```python
from build123d import *

# Parameters (mm, degrees)
F1_DEPTH = 18
F2_R     = 3
F3_R     = 3
F4_R     = 12
F5_R     = 0.5


with BuildPart() as f1:
    # F0 (on Top) → F1 (new body)
    with BuildSketch(Plane.XY):
        Polygon((-61.901969, -15.611527), (28.098031, -15.611527), (20.267047, 16.256898), (12.498162, 14.347861), (17.032125, -4.103242), (7.746533, -3.611527), (-6.571248, 54.655111), (-14.340133, 52.746074), (0, -5.611527), (-61.901969, -5.611527), align=None)
    extrude(amount=F1_DEPTH)

    # F2
    f2_edges = [f1.edges().sort_by_distance(p)[0] for p in [
        (12.498162, 14.347861, 9),
        (-6.571248, 54.655111, 9),
    ]]
    fillet(f2_edges, radius=F2_R)

    # F3
    f3_edges = [f1.edges().sort_by_distance(p)[0] for p in [
        (-61.901969, -5.611527, 9),
    ]]
    fillet(f3_edges, radius=F3_R)

    # F4
    f4_edges = [f1.edges().sort_by_distance(p)[0] for p in [
        (0, -5.611527, 9),
    ]]
    fillet(f4_edges, radius=F4_R)

    # F5
    f5_edges = [f1.edges().sort_by_distance(p)[0] for p in [
        (17.032125, -4.103242, 9),
        (7.746533, -3.611527, 9),
    ]]
    fillet(f5_edges, radius=F5_R)


solid = f1.part
```
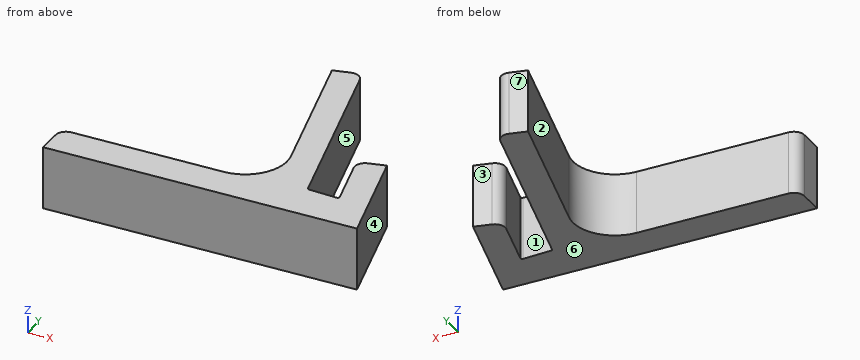
Geometry check sheet. Reference: the model listing, model coordinates, mm. Face numbers are marked on the shaded views. A direction names the side the tool comes from. Coordinates: 2 decimals unless noted, no trailing zeros. Order: outer loops, then holes, each group sorted by start corner. A loop starts at its lowest first (then second) coordinate and runs counter-clockwise, first axis right, second up.
Item 1: Scan lines: line 1 along Y through (x, z) = (8.5, 14); line 2 along Y through (x, z) = (-31, 17); line 3 along X through (y, z) = (-3.5, 6). Record each from-to range of solid material in increasing order.
Item 2: Section check B-B (z = 10.75). Enter the section's corners in (x, y).
Item 3: Section check A-A (y = 2.5). Enter the section's corners in (x, z), plus the area to 3 significant figures.
Item 4: Depth check by flat-ended pin: pin 1 (2 mm diameter, centred on x = -32.5, z = 11.5, fed in from +Y); pin 2 (1 mm diameter, centred on y = 31, z = 13, fed in from +X). Enter the tip coordinate at first touch or a pass-through.
Item 5: Section check C-C (x = -34). Enter the section's corners in (y, z), plus the area to 3 significant figures.
Item 6: Mould release check, pull along X, two halves, no side actions. Record for the marked faces 4, 5, 6 and 7: released by +X, released by -X, zero draft, split by the parting line, or undercut.
Item 7: Tool access check on the marked faces 1, 2 and 3. Record the directions out of +Z, -Z, +X, -X, +Y, -Y that give a thin tool (end or side, any length) a straight path to the whole face; none if there is none.
Item 8: Section check D-D (y = 28.5). Enter the section's corners in (x, z), plus the area to 3 significant figures.
Check sheet entries:
1. line 1: y = -15.61 to -3.65
1. line 2: y = -15.61 to -5.61
1. line 3: x = -8.51 to 7.81, 16.88 to 25.12
2. outline: (-61.9, -15.61) - (28.1, -15.61) - (20.27, 16.26) - (15.41, 15.06) arc R3 ccw to (13.21, 11.43) - (16.87, -3.45) arc R0.5 cw to (16.36, -4.07) - (8.12, -3.63) arc R0.5 cw to (7.66, -3.25) - (-5.86, 51.74) arc R3 ccw to (-9.48, 53.94) - (-14.34, 52.75) - (-3.65, 9.25) arc R12 cw to (-15.31, -5.61) - (-58.9, -5.61) arc R3 ccw to (-61.9, -8.61) - close
3. outline: (-3.95, 0) - (6.24, 0) - (6.24, 18) - (-3.95, 18) - close; (15.41, 0) - (23.65, 0) - (23.65, 18) - (15.41, 18) - close
3. area: 332 mm2
4. pin 1: stops at y = -5.61
4. pin 2: stops at x = -0.64
5. outline: (-15.61, 0) - (-5.61, 0) - (-5.61, 18) - (-15.61, 18) - close
5. area: 180 mm2
6. face 4: released by +X
6. face 5: undercut
6. face 6: zero draft
6. face 7: released by -X
7. face 1: +Z, -Z
7. face 2: +Z, -Z, -X
7. face 3: +Z, -Z, +Y
8. outline: (-8.38, 0) - (-0.14, 0) - (-0.14, 18) - (-8.38, 18) - close
8. area: 148 mm2
